Source: CAD feature listing. Evaluate the final solid. Frame: model axes, mm. Face numbers are marked on the shaded views. A direction names the side the tool comes from. Round coordinates to 2 decimals unless told otherwise and drop trailing zeros. Order: outer loops, then holes, each group sorted by start corner. A loop starts at its lowest first (then second) coordinate and runs counter-clockwise, first axis right, second up. Notation, with made-up numbers: M 79,89 L 138,89 A16 cw 138,117 Z; hole C 49,-23.5 d6. An arc over 180 degrees is marked long. Use one line per item in the form item = value. Start each with the question number.
Q1. Section A-A (y = -32.5). Return the cut outline in (x, z), plus the area to 3 significant figures.
Q2. Reachability of the marked faces 1 and 2 from +Z, -Z, +X, -X, +Y, -Y: full face, straight path, thin tool, end or side. Return the list, or none.
Q3. Section C-C (x = 0). Return the cut outline in (y, z), plus the area to 3 significant figures.
Q4. Section B-B (z = 150). Return the cut outline in (x, y).
Q5. Contact query for flat-ended pins moving along their axis: pin 1 (1.5 mm diameter, centred on x = 1, z = 141.5, fed in from +Y); pin 2 (12 mm diameter, centred on x = -15.5, z = 158, fed in from +Y); pin 3 (4 mm diameter, centred on x = -3.5, y = 9, fed in from +Z). Output: stop coordinate, or through.
Q6. Section D-D (x = -6). Return the cut outline in (y, z).
Q7. Material intervals for probe 1 along Y at (x, z) = (-16.5, 147); probe 2 along Z at (x, y) = (-19, -41.5), sorted ascending.
from build123d import *

# Parameters (mm, degrees)
SKETCH045_W             = 42.5
SKETCH045_H             = 42.5
PAD015_DEPTH            = 47.4
CHAMFER009_SIZE         = 5
CHAMFER008_SIZE         = 5
CHAMFER010_SIZE         = 5
CHAMFER011_SIZE         = 5
SKETCH047_R             = 11
PAD016_DEPTH            = 1.5
SKETCH046_R             = 2.5
PAD014_DEPTH            = 18.5
BODY010_PLACEMENT_ANGLE = 180


with BuildPart() as part:
    # Sketch045 → Pad015 (new body)
    with BuildSketch(Plane.XZ):
        Rectangle(SKETCH045_W, SKETCH045_H)
    extrude(amount=-PAD015_DEPTH)

    # Chamfer009
    chamfer009_edges = [part.edges().sort_by_distance(p)[0] for p in [
        (21.25, 23.7, 21.25),
    ]]
    chamfer(chamfer009_edges, length=CHAMFER009_SIZE)

    # Chamfer008
    chamfer008_edges = [part.edges().sort_by_distance(p)[0] for p in [
        (-21.25, 23.7, 21.25),
    ]]
    chamfer(chamfer008_edges, length=CHAMFER008_SIZE)

    # Chamfer010
    chamfer010_edges = [part.edges().sort_by_distance(p)[0] for p in [
        (21.25, 23.7, -21.25),
    ]]
    chamfer(chamfer010_edges, length=CHAMFER010_SIZE)

    # Chamfer011
    chamfer011_edges = [part.edges().sort_by_distance(p)[0] for p in [
        (-21.25, 23.7, -21.25),
    ]]
    chamfer(chamfer011_edges, length=CHAMFER011_SIZE)

    # Sketch047 (on Face1 of Chamfer011) → Pad016 (join)
    with BuildSketch(Plane.XZ):
        Circle(SKETCH047_R)
    extrude(amount=PAD016_DEPTH)

    # Sketch046 (on Face12 of Pad016) → Pad014 (join)
    with BuildSketch(Plane.XZ.offset(1.5)):
        Circle(SKETCH046_R)
    extrude(amount=PAD014_DEPTH)


with BuildPart() as part_1:
    # Body010 placement: moved
    add(part.part.moved(Location((0, -2.25, 150))).rotate(Axis((0, -2.25, 150), (0, 0, 1)), BODY010_PLACEMENT_ANGLE))


solid = part_1.part
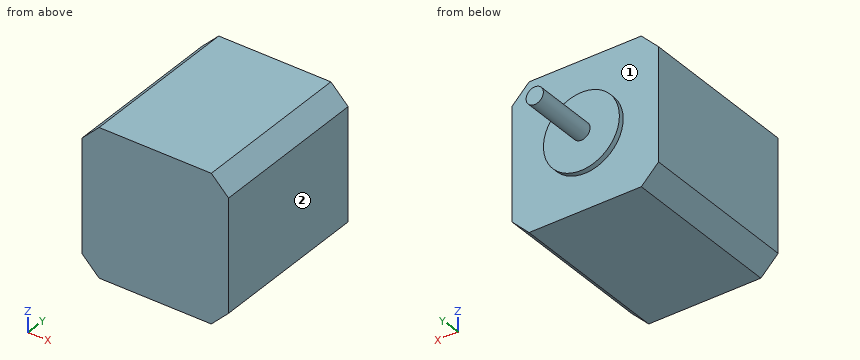
Results list:
q1.outline = M -21.25,133.75 L -16.25,128.75 L 16.25,128.75 L 21.25,133.75 L 21.25,166.25 L 16.25,171.25 L -16.25,171.25 L -21.25,166.25 Z
q1.area = 1,760 mm2
q2.face_1 = +Y
q2.face_2 = +Z, -Z, +X, +Y, -Y
q3.outline = M -49.65,128.75 L -2.25,128.75 L -2.25,139 L -0.75,139 L -0.75,147.5 L 17.75,147.5 L 17.75,152.5 L -0.75,152.5 L -0.75,161 L -2.25,161 L -2.25,171.25 L -49.65,171.25 Z
q3.area = 2,140 mm2
q4.outline = M -21.25,-49.65 L 21.25,-49.65 L 21.25,-2.25 L 11,-2.25 L 11,-0.75 L 2.5,-0.75 L 2.5,17.75 L -2.5,17.75 L -2.5,-0.75 L -11,-0.75 L -11,-2.25 L -21.25,-2.25 Z
q5.pin_1 = -0.75
q5.pin_2 = -2.25
q5.pin_3 = 152
q6.outline = M -49.65,128.75 L -2.25,128.75 L -2.25,140.78 L -0.75,140.78 L -0.75,159.22 L -2.25,159.22 L -2.25,171.25 L -49.65,171.25 Z
q7.probe_1 = -49.65 to -2.25
q7.probe_2 = 131.5 to 168.5
